```python
from build123d import *

# Parameters (mm, degrees)
BOSS_EXTRU_1_DEPTH      = 7
ESQUISSE2_R             = 3.125
ENL_V_MAT_EXTRU_1_DEPTH = 7
ENL_V_MAT_EXTRU_2_DEPTH = 6
ENL_V_MAT_EXTRU_3_REACH = 102.076
ESQUISSE4_W             = 8
ESQUISSE4_H             = 4
CHANFREIN1_SIZE         = 2
ESQUISSE5_R             = 1
ENL_V_MAT_EXTRU_4_DEPTH = 110.041839956
ESQUISSE7_R             = 1.5
ENL_V_MAT_EXTRU_6_DEPTH = 8


with BuildPart() as part:
    # Esquisse1 → Boss.-Extru.1 (new body)
    with BuildSketch(Plane(origin=(0, 0, 0), x_dir=(1, 0, 0), z_dir=(0, 1, 0))):
        with BuildLine():
            Line((-71.649484536, 25), (-31.649484536, 25))
            ThreePointArc((-31.649484536, 25), (-6.649484536, 0), (-31.649484536, -25))
            Line((-31.649484536, -25), (-71.649484536, -25))
            ThreePointArc((-71.649484536, -25), (-96.649484536, 0), (-71.649484536, 25))
        make_face()
    extrude(amount=BOSS_EXTRU_1_DEPTH)

    # Esquisse2 → Enlèv. mat.-Extru.1 (cut)
    with BuildSketch(Plane(origin=(0, 7, 0), x_dir=(1, 0, 0), z_dir=(0, 1, 0))):
        with Locations(Location((-71.649484536, 0, 0), (0, 0, 270))):
            Circle(ESQUISSE2_R)
    extrude(amount=-ENL_V_MAT_EXTRU_1_DEPTH, mode=Mode.SUBTRACT)

    # Esquisse3 → Enlèv. mat.-Extru.2 (cut)
    with BuildSketch(Plane(origin=(0, 7, 0), x_dir=(1, 0, 0), z_dir=(0, 1, 0))):
        Polygon((-51.649484536, 30.5), (-27.149484536, 30.5), (-27.149484536, 14), (-23.149484536, 14), (-23.149484536, 12), (-27.149484536, 12), (-27.149484536, -1.5), (-51.649484536, -1.5), (-51.649484536, 12), (-55.649484536, 12), (-55.649484536, 14), (-51.649484536, 14), align=None)
    extrude(amount=-ENL_V_MAT_EXTRU_2_DEPTH, mode=Mode.SUBTRACT)

    # Esquisse4 → Enlèv. mat.-Extru.3 (cut, up to next)
    with BuildSketch(Plane(origin=(0, 7, 0), x_dir=(1, 0, 0), z_dir=(0, 1, 0)), mode=Mode.PRIVATE) as enl_v_mat_extru_3_sk1:
        with Locations((-61.649484536, 0)):
            Rectangle(ESQUISSE4_W, ESQUISSE4_H)
    enl_v_mat_extru_3_tool1 = extrude(enl_v_mat_extru_3_sk1.sketch, amount=-ENL_V_MAT_EXTRU_3_REACH, mode=Mode.PRIVATE) & part.part
    add(enl_v_mat_extru_3_tool1.solids().sort_by_distance((-61.649485, 7, 0))[0], mode=Mode.SUBTRACT)

    # Chanfrein1
    chanfrein1_edges = [part.edges().sort_by_distance(p)[0] for p in [
        (-57.649484536, 7, 0),
    ]]
    chamfer(chanfrein1_edges, length=CHANFREIN1_SIZE)

    # Esquisse5 → Enlèv. mat.-Extru.4 (cut, through all)
    with BuildSketch(Plane.XY.offset(25)):
        with Locations((-61.649484536, 3.5)):
            Circle(ESQUISSE5_R)
    extrude(amount=-ENL_V_MAT_EXTRU_4_DEPTH, mode=Mode.SUBTRACT)

    # Esquisse7 → Enlèv. mat.-Extru.6 (cut)
    with BuildSketch(Plane(origin=(0, 7, 0), x_dir=(1, 0, 0), z_dir=(0, 1, 0))):
        with Locations(Location((-16.649484536, 0, 0), (0, 0, 270))):
            Circle(ESQUISSE7_R)
        with Locations(Location((-82.963193035, 11.313708499, 0), (0, 0, 270))):
            Circle(ESQUISSE7_R)
        with Locations(Location((-82.963193035, -11.313708499, 0), (0, 0, 270))):
            Circle(ESQUISSE7_R)
        with Locations(Location((-61.399484536, 13, 0), (0, 0, 270))):
            Circle(ESQUISSE7_R)
        with Locations(Location((-17.399484536, 13, 0), (0, 0, 270))):
            Circle(ESQUISSE7_R)
    extrude(amount=-ENL_V_MAT_EXTRU_6_DEPTH, mode=Mode.SUBTRACT)


solid = part.part
```
Can you work these out from the model? Positions are in its coordinate system, mm. A direction names the side the tool comes from. Round coordinates to 2 decimals unless told otherwise and drop trailing zeros. Loops run counter-clockwise (first coordinate to the right, second up) from the corner with the lowest first, then second, coordinate; pieces in that order, holes last. Notation, with made-up numbers: M -13,6 L 6,6 A29 cw 6,45 Z; hole C 54,-23.5 d4. An arc over 180 degrees is marked long. Write item = value, one per line. Start each with the question number.
(1) Which directions (+Z, -Z, +X, -X, +Y, -Y) give clear straight access to the entire face, cutting with the end or side of a thin tool? Please do faces 1 (the face through (-27.149, 4, -19)), 2 (the face through (-23.149, 4, -13)), 3 (the face through (-65.649, 4, 0)).
(2) I'm going to push flat-ended pins straight in: P1, Ø3, axis at x = -25.5, y = 3.5, coming from the +Z side; P2, Ø2, axis at y = 3, z = -13.5, coming from the +X side; P3, Ø3, axis at x = -24.5, y = 3, coming from the -Z side; P4, Ø10, axis at x = -71.65, z = 0, coming from the -Y side. Where does each tip first touch, or does it pass through?
(3) Suppose I cut it at A-A on z = 0. Write out the boundary of the cut face in (x, y), plus the area to 3 significant figures.
(4) Suppose I cut it at C-C on y = 3.5. Give the number of separate pieces and of enclosed holes in the cut face, plus the area to 3 significant figures.
(5) I need wall thicknesses on line 1 along Z through (x, y) = (-53, 5.75); line 2 along X through (y, z) = (3.5, -4.25); line 3 along X through (y, z) = (5.5, -13). Which ranges of each line are inside material? Lowest first, please.
(6) If we mould it in two halves opening along Z, with no side actions, what happens to faces 4 (the face through (-74.422, 3.549, 1.442)), 5 (the face through (-96.643, 3.451, 0.55)), 6 (the face through (-51.649, 4, -5))? For each: released by +Z, released by -Z, zero draft, split by the parting line, or undercut.
(7) Suppose I cut it at D-D on z = 17.5. Write out the boundary of the cut face in (x, y), plus the area to 3 significant figures.
(8) Suppose I cut it at B-B on x = -39.5. Write out the boundary of the cut face in (y, z), plus the area to 3 significant figures.
Answer block:
q1.face_1 = -Z, +Y
q1.face_2 = +Y
q1.face_3 = +Y, -Y
q2.P1 = 24.56
q2.P2 = -10
q2.P3 = -24.35
q2.P4 = 0
q3.outline = M -96.65,0 L -74.77,0 L -74.77,7 L -96.65,7 Z; M -68.52,0 L -65.65,0 L -65.65,7 L -68.52,7 Z; M -57.65,0 L -18.15,0 L -18.15,7 L -27.15,7 L -27.15,1 L -51.65,1 L -51.65,7 L -55.65,7 L -57.65,5 Z; M -15.15,0 L -6.65,0 L -6.65,7 L -15.15,7 Z
q3.area = 360 mm²
q4.separate_pieces = 2
q4.enclosed_holes = 5
q4.area = 3,110 mm²
q5.line_1 = -25 to -14, -12 to 25
q5.line_2 = -96.29 to -62.65, -60.65 to -51.65, -27.15 to -7.01
q5.line_3 = -93 to -62.9, -59.9 to -55.65, -23.15 to -18.9, -15.9 to -10.3
q6.face_4 = undercut
q6.face_5 = split by the parting line
q6.face_6 = zero draft
q7.outline = M -89.5,0 L -13.8,0 L -13.8,7 L -89.5,7 Z; hole C -61.65,3.5 d2
q7.area = 527 mm²
q8.outline = M 0,-25 L 1,-25 L 1,1.5 L 7,1.5 L 7,25 L 0,25 Z
q8.area = 191 mm²
